Input: part model. Units: mm. Frame: model coordinates. A direction names the side the tool comes from. Give positions to 0.01 mm unless a question says otherwise; leave off trailing zeros. Return JSON: item names as keys, results as strings. Group by question number.
Item 1: Line query: line 1 (X direction, y = 6.5, z = 3.85); line 2 (Y direction, x = -7, z = 3.4); line 3 (Z direction, x = 3.25, y = -2.25). Output: solid intervals per line, ascending. Write a range as [from, to].
Item 2: Set-up query: faces 1 (the face through (0.37, 7.26, 2.22)), 2 (the face through (4.867, -5.394, 2.218)), 3 (the face through (-7.28, -0.36, 2.22)), 4 (the face through (7.28, 0.36, 2.22)). Return all of +Z, -Z, +X, -X, +Y, -Y with unobstructed straight access to the full face (end or side cutting, diameter ignored); none if empty.
Item 3: Mould query, pull axis X, two halves, no side actions, for faces 5 (the face through (0, -6, 4.5)), 6 (the face through (1.518, -7.104, 2.22)), 7 (the face through (6.48, -3.32, 2.22)). Classes: released by +X, released by -X, zero draft, split by the parting line, or undercut.
Item 4: Pin query (flat end, axial travel): P1, Ø4, axis at x = -5.5, y = 5.5, coming from the -Z side; P2, Ø1, axis at x = 6.5, z = 4, coming from the +Y side; P3, Ø1.5, axis at y = -4, z = 3, coming from the -X side; P4, Ø5.5, axis at x = 0, y = 0, coming from the -Z side. Return the tip coordinate at first contact, or that it passes through.
from build123d import *

# Parameters (mm, degrees)
F0_R     = 5.5
F1_DEPTH = 4.5
F0_R_2   = 3.15
F2_DEPTH = 1.3
F3_R     = 0.2
F4_R     = 0.1


with BuildPart() as f1:
    # F0 (on Top) → F1 (new body)
    with BuildSketch(Plane.XY):
        with BuildLine():
            ThreePointArc((0.980887, 6.498578), (0.849077, 6.449381), (0.734492, 6.531016))
            Line((0.734492, 6.531016), (0, 8))
            Line((0, 8), (-0.734492, 6.531016))
            ThreePointArc((-0.734492, 6.531016), (-0.849077, 6.449381), (-0.980887, 6.498578))
            Line((-0.980887, 6.498578), (-2.070552, 7.727407))
            Line((-2.070552, 7.727407), (-2.399816, 6.118376))
            ThreePointArc((-2.399816, 6.118376), (-2.489368, 6.009867), (-2.629419, 6.023272))
            Line((-2.629419, 6.023272), (-4, 6.928203))
            Line((-4, 6.928203), (-3.901597, 5.28878))
            ThreePointArc((-3.901597, 5.28878), (-3.960013, 5.160789), (-4.098761, 5.13749))
            Line((-4.098761, 5.13749), (-5.656854, 5.656854))
            Line((-5.656854, 5.656854), (-5.13749, 4.098761))
            ThreePointArc((-5.13749, 4.098761), (-5.160789, 3.960013), (-5.28878, 3.901597))
            Line((-5.28878, 3.901597), (-6.928203, 4))
            Line((-6.928203, 4), (-6.023272, 2.629419))
            ThreePointArc((-6.023272, 2.629419), (-6.009867, 2.489368), (-6.118376, 2.399816))
            Line((-6.118376, 2.399816), (-7.727407, 2.070552))
            Line((-7.727407, 2.070552), (-6.498578, 0.980887))
            ThreePointArc((-6.498578, 0.980887), (-6.449381, 0.849077), (-6.531016, 0.734492))
            Line((-6.531016, 0.734492), (-8, 0))
            Line((-8, 0), (-6.531016, -0.734492))
            ThreePointArc((-6.531016, -0.734492), (-6.449381, -0.849077), (-6.498578, -0.980887))
            Line((-6.498578, -0.980887), (-7.727407, -2.070552))
            Line((-7.727407, -2.070552), (-6.118376, -2.399816))
            ThreePointArc((-6.118376, -2.399816), (-6.009867, -2.489368), (-6.023272, -2.629419))
            Line((-6.023272, -2.629419), (-6.928203, -4))
            Line((-6.928203, -4), (-5.28878, -3.901597))
            ThreePointArc((-5.28878, -3.901597), (-5.160789, -3.960013), (-5.13749, -4.098761))
            Line((-5.13749, -4.098761), (-5.656854, -5.656854))
            Line((-5.656854, -5.656854), (-4.098761, -5.13749))
            ThreePointArc((-4.098761, -5.13749), (-3.960013, -5.160789), (-3.901597, -5.28878))
            Line((-3.901597, -5.28878), (-4, -6.928203))
            Line((-4, -6.928203), (-2.629419, -6.023272))
            ThreePointArc((-2.629419, -6.023272), (-2.489368, -6.009867), (-2.399816, -6.118376))
            Line((-2.399816, -6.118376), (-2.070552, -7.727407))
            Line((-2.070552, -7.727407), (-0.980887, -6.498578))
            ThreePointArc((-0.980887, -6.498578), (-0.849077, -6.449381), (-0.734492, -6.531016))
            Line((-0.734492, -6.531016), (0, -8))
            Line((0, -8), (0.734492, -6.531016))
            ThreePointArc((0.734492, -6.531016), (0.849077, -6.449381), (0.980887, -6.498578))
            Line((0.980887, -6.498578), (2.070552, -7.727407))
            Line((2.070552, -7.727407), (2.399816, -6.118376))
            ThreePointArc((2.399816, -6.118376), (2.489368, -6.009867), (2.629419, -6.023272))
            Line((2.629419, -6.023272), (4, -6.928203))
            Line((4, -6.928203), (3.901597, -5.28878))
            ThreePointArc((3.901597, -5.28878), (3.960013, -5.160789), (4.098761, -5.13749))
            Line((4.098761, -5.13749), (5.656854, -5.656854))
            Line((5.656854, -5.656854), (5.13749, -4.098761))
            ThreePointArc((5.13749, -4.098761), (5.160789, -3.960013), (5.28878, -3.901597))
            Line((5.28878, -3.901597), (6.928203, -4))
            Line((6.928203, -4), (6.023272, -2.629419))
            ThreePointArc((6.023272, -2.629419), (6.009867, -2.489368), (6.118376, -2.399816))
            Line((6.118376, -2.399816), (7.727407, -2.070552))
            Line((7.727407, -2.070552), (6.609232, -1.079009))
            ThreePointArc((6.609232, -1.079009), (6.527238, -0.859327), (6.663296, -0.668352))
            Line((6.663296, -0.668352), (8, 0))
            Line((8, 0), (6.531016, 0.734492))
            ThreePointArc((6.531016, 0.734492), (6.449381, 0.849077), (6.498578, 0.980887))
            Line((6.498578, 0.980887), (7.727407, 2.070552))
            Line((7.727407, 2.070552), (5.973485, 2.429466))
            ThreePointArc((5.973485, 2.429466), (5.937315, 2.459317), (5.941784, 2.506))
            Line((5.941784, 2.506), (6.928203, 4))
            Line((6.928203, 4), (5.28878, 3.901597))
            ThreePointArc((5.28878, 3.901597), (5.160789, 3.960013), (5.13749, 4.098761))
            Line((5.13749, 4.098761), (5.656854, 5.656854))
            Line((5.656854, 5.656854), (4.098761, 5.13749))
            ThreePointArc((4.098761, 5.13749), (3.960013, 5.160789), (3.901597, 5.28878))
            Line((3.901597, 5.28878), (4, 6.928203))
            Line((4, 6.928203), (2.629419, 6.023272))
            ThreePointArc((2.629419, 6.023272), (2.489368, 6.009867), (2.399816, 6.118376))
            Line((2.399816, 6.118376), (2.070552, 7.727407))
            Line((2.070552, 7.727407), (0.980887, 6.498578))
        make_face()
        Circle(F0_R, mode=Mode.SUBTRACT)
    extrude(amount=F1_DEPTH)

    # F0 (on Top) → F2 (join)
    with BuildSketch(Plane.XY):
        Circle(F0_R)
        Circle(F0_R_2, mode=Mode.SUBTRACT)
    extrude(amount=F2_DEPTH)

    # F3
    f3_edges = [f1.edges().sort_by_distance(p)[0] for p in [
        (-3.15, 0, 1.3),
        (-5.5, 0, 1.3),
        (-5.5, 0, 4.5),
        (-3.15, 0, 0),
    ]]
    fillet(f3_edges, radius=F3_R)

    # F4
    f4_edges = [f1.edges().sort_by_distance(p)[0] for p in [
        (0.367246, -7.265508, 4.5),
        (0.367246, -7.265508, 0),
    ]]
    fillet(f4_edges, radius=F4_R)


solid = f1.part
Answer below:
{
 "1": {"line 1": "x = [-3.97, -3.35], [-2.32, -0.98], [-0.76, 0.76], [0.98, 2.32], [3.35, 3.97]", "line 2": "y = [-2.22, -1.43], [-0.5, 0.5], [1.43, 2.22]", "line 3": "z = [0, 1.3]"},
 "2": {"face 1": "+Z, -Z, +Y", "face 2": "+Z, -Z, -Y", "face 3": "+Z, -Z, -X", "face 4": "+Z, -Z, +X"},
 "3": {"face 5": "zero draft", "face 6": "undercut", "face 7": "released by +X"},
 "4": {"P1": "stops at z = 0", "P2": "stops at y = 4", "P3": "stops at x = -6.93", "P4": "passes through"}
}
